Check sheet for the modelled part. Datum: model origin and axes. Units: mm. Face numbers are marked on the shaded views. A direction names the side the tool comes from. Give positions to 0.01 mm unless a question says otherwise; leave off trailing zeros. Loops run counter-clockwise (first coordinate to the right, second up) from the corner with the lowest first, then second, coordinate; pieces in that order, holes last. Notation, with made-up numbers: M 17.5,-22 L 66.5,-22 A17 cw 66.5,8 Z; hole C 50,53 d5. An arc over 180 degrees is marked long. Use one line per item in the form item = value.
from build123d import *

# Parameters (mm, degrees)
F0_W     = 165.1
F0_H     = 82.55
F0_R     = 17.4625
F0_W_2   = 25.4
F1_DEPTH = 19.05
F2_DEPTH = 57.15
F4_DEPTH = 25.4
F3_R     = 17.4625
F5_DEPTH = 25.4


with BuildPart() as f1:
    # F0 (on Top) → F1 (new body)
    with BuildSketch(Plane.XY):
        with Locations((12.7, 0)):
            Rectangle(F0_W, F0_H)
        with Locations((-19.05, 0)):
            Circle(F0_R, mode=Mode.SUBTRACT)
        with Locations((57.15, 0)):
            Circle(F0_R, mode=Mode.SUBTRACT)
        with Locations((-82.55, 0)):
            Rectangle(F0_W_2, F0_H)
    extrude(amount=F1_DEPTH)

    # F0 (on Top) → F2 (join)
    with BuildSketch(Plane.XY):
        with Locations((-82.55, 0)):
            Rectangle(F0_W_2, F0_H)
    extrude(amount=F2_DEPTH)

    # F3 (on face) → F4 (join)
    with BuildSketch(Plane.YZ.offset(-69.85)):
        with BuildLine():
            ThreePointArc((-17.4625, 57.15), (0, 74.6125), (17.4625, 57.15))
            Line((17.4625, 57.15), (41.275, 57.15))
            ThreePointArc((41.275, 57.15), (0, 98.425), (-41.275, 57.15))
            Line((-41.275, 57.15), (-17.4625, 57.15))
        make_face()
    extrude(amount=-F4_DEPTH)

    # F3 (on face) → F5 (cut)
    with BuildSketch(Plane.YZ.offset(-69.85)):
        with Locations((0, 57.15)):
            Circle(F3_R)
    extrude(amount=-F5_DEPTH, mode=Mode.SUBTRACT)


solid = f1.part
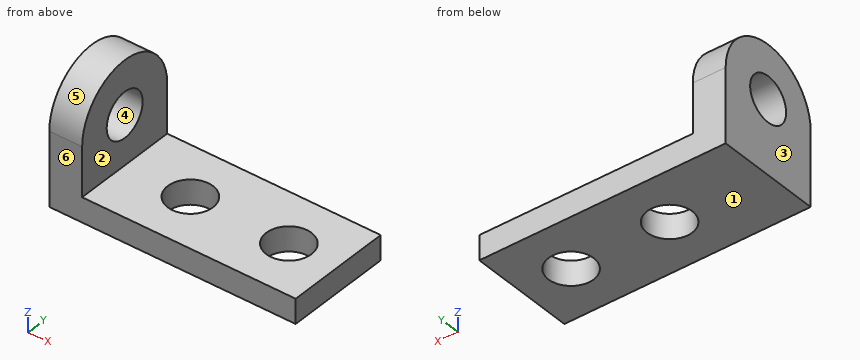
1) Section check C-C (y = -23). Record the cut outline in (x, z).
Evaluation:
outline = M -95.25,0 L 95.25,0 L 95.25,19.05 L -69.85,19.05 L -69.85,91.42 L -95.25,91.42 Z
2) Set-up check for the marked faces 1 and 2: record each of +Z, -Z, +X, -X, +Y, -Y from which the full face is reachable in a straight line by a thin tool's end or side.
Evaluation:
face_1 = -Z, +X, -X, +Y, -Y
face_2 = +Z, +X, +Y, -Y
3) Depth check by flat-ended pin: pin 1 Ø25 at (x, y) = (51.5, -1) entering from +Z; pin 2 Ø21 at (x, y) = (-19.05, 0) entering from -Z; pin 3 Ø4 at (y, z) = (22, 60) entering from +X. Enter the tip coordinate at first touch or a pass-through.
Evaluation:
pin_1 = 19.05
pin_2 = through
pin_3 = -69.85
4) Release check for a two-part mould opening along Y. For the marked faces 3, 4, 5 and 6 record: pulls with the +Y half, pulls with the -Y half, needs draft (parallel to the pull), parting line crosses it, or undercut.
Evaluation:
face_3 = needs draft
face_4 = undercut
face_5 = parting line crosses it
face_6 = pulls with the -Y half
5) Section check A-A (y = 0). State how many separate pieces and enclosed holes the cut face has, then the cut area to 3 significant figures.
Evaluation:
separate_pieces = 4
enclosed_holes = 0
area = 3,430 mm^2
6) Section check D-D (x = 9.5). Record the cut outline in (y, z) (3 decimals), then the cut area to 3 significant figures.
Evaluation:
outline = M -41.275,0 L 41.275,0 L 41.275,19.05 L -41.275,19.05 Z
area = 1,570 mm^2
7) Scan lines: line 1 (Y direction, x = 57.15, z = 10.25) (1 decimal); line 2 (X direction, y = -13, z = 11); line 3 (Z direction, x = -85, y = 0) (1 decimal). Record each from-to range of solid material in increasing order.
Evaluation:
line_1 = -41.3 to -17.5, 17.5 to 41.3
line_2 = -95.25 to -30.71, -7.39 to 45.49, 68.81 to 95.25
line_3 = 0 to 39.7, 74.6 to 98.4
